from build123d import *

# Parameters (mm, degrees)
SKETCH1_R           = 1.905
BOSS_EXTRUDE1_DEPTH = 2.54
FILLET5_R           = 5.08
FILLET6_R           = 2.54


with BuildPart() as part:
    # Sketch1 → Boss-Extrude1 (new body)
    with BuildSketch(Plane.XY):
        with BuildLine():
            Line((5.08, 10.16), (7.62, 12.7))
            Line((7.62, 12.7), (50.8, 12.7))
            Line((50.8, 12.7), (50.8, -2.54))
            Line((50.8, -2.54), (50.8, -8.255))
            ThreePointArc((50.8, -8.255), (48.895, -10.16), (50.8, -12.065))
            Line((50.8, -12.065), (50.8, -15.24))
            ThreePointArc((50.8, -15.24), (47.896976236, -14.328795153), (46.035389215, -11.922068121))
            Line((46.035389215, -11.922068121), (44.38107747, -2.54))
            Line((44.38107747, -2.54), (7.62, -2.54))
            Line((7.62, -2.54), (5.08, 0))
            Line((5.08, 0), (0, 0))
            Line((0, 0), (0, 10.16))
            Line((0, 10.16), (5.08, 10.16))
        make_face()
        with Locations((5.08, 5.08)):
            Circle(SKETCH1_R, mode=Mode.SUBTRACT)
    extrude(amount=BOSS_EXTRUDE1_DEPTH)

    # Fillet5
    fillet5_edges = [part.edges().sort_by_distance(p)[0] for p in [
        (44.38107747, -2.54, 1.27),
        (0, 0, 1.27),
        (0, 10.16, 1.27),
    ]]
    fillet(fillet5_edges, radius=FILLET5_R - 0.0001)  # a hair under: the kernel refuses the full size

    # Fillet6
    fillet6_edges = [part.edges().sort_by_distance(p)[0] for p in [
        (5.08, 10.16, 1.27),
        (7.62, 12.7, 1.27),
        (7.62, -2.54, 1.27),
        (5.08, 0, 1.27),
    ]]
    fillet(fillet6_edges, radius=FILLET6_R)

    # Mirror5: part across plane


with BuildPart() as part_1:
    add(part.part)
    add(part.part.mirror(Plane(origin=(50.8, -2.54, 2.54), x_dir=(0, 0, 1), z_dir=(-1, 0, 0))))


solid = part_1.part
CAD build for the part. Positions are in the model's coordinates, mm. A direction names the side the tool comes from. Coordinates: 2 decimals unless noted, no trailing zeros. Loops run counter-clockwise (first coordinate to the right, second up) from the corner with the lowest first, then second, coordinate; pieces in that order, holes last. Notation, with made-up numbers: (-27.75, 4) -> (24.25, 4) arc R17 cw to (24.25, 31) -> close; hole circle Ø7 at (75, -25.75). An arc over 180 degrees is marked (long way). One line per item, written item: value.
1. Slice it at A-A on y = -10.16. Write the cut outline in (x, z) (3 decimals), and give its area (3 significant figures).
Answers:
outline: (45.725, 0) -> (48.895, 0) -> (48.895, 2.54) -> (45.725, 2.54) -> close; (52.705, 0) -> (55.875, 0) -> (55.875, 2.54) -> (52.705, 2.54) -> close
area: 16.1 mm^2
2. Slice it at B-B on x = 38. Write the cut outline in (y, z).
Answers:
outline: (-2.54, 0) -> (12.7, 0) -> (12.7, 2.54) -> (-2.54, 2.54) -> close
3. Flat gauge pins, fed straight in: P1, Ø0.8, axis at x = 81, z = 2, coming from the -Y side; P2, Ø1, axis at y = 0.5, z = 1.5, coming from the -X side. Where does each tip first touch, or does it go through?
Answers:
P1: stops at y = -2.54
P2: stops at x = 2.05
4. Which spindle directions (+Z, -Z, +X, -X, +Y, -Y) get a long thin tool onto all of the face, cutting with end or side? Do faces 5 (the face through (25, -2.54, 1)), 6 (the face through (77, -2.54, 1)), 7 (the face through (51, 12.7, 1)). Say none if no direction does.
Answers:
face 5: +Z, -Z, -X, -Y
face 6: +Z, -Z, +X, -Y
face 7: +Z, -Z, +X, -X, +Y
5. Slice it at C-C on z = 1. Give the number of separate pieces and of enclosed holes in the cut face, and give its area (3 significant figures).
Answers:
separate pieces: 1
enclosed holes: 3
area: 1,560 mm^2
6. Drill centre lines: line 1 (X direction, y = 4, z = 0.2); line 2 (X direction, y = 5.75, z = 0.9); line 3 (Y direction, x = 93, z = 1.1). Where is each one in solid material? Low to high. Write a range as [from, to].
Answers:
line 1: x = [0.12, 3.51], [6.65, 94.95], [98.09, 101.48]
line 2: x = [0.04, 3.3], [6.86, 94.74], [98.3, 101.56]
line 3: y = [-2.54, 12.7]
7. Slice it at D-D on y = 8.25. Write the cut outline in (x, z), and give its area (3 significant figures).
Answers:
outline: (1.11, 0) -> (100.49, 0) -> (100.49, 2.54) -> (1.11, 2.54) -> close
area: 252 mm^2
8. Pull direction X, two halves, no side cores. Call faces 1 (the face through (56.015, -9.366, 1.252)), 2 (the face through (50, 5, 0)), 3 (the face through (3.57, 3.92, 1.25)), 4 (the face through (98.423, 5.164, 1.252)): pulls with the +X half, pulls with the -X half, needs draft (parallel to the pull), parting line crosses it, or undercut.
Answers:
face 1: pulls with the +X half
face 2: needs draft
face 3: undercut
face 4: undercut
